Can you work these out from the drawing? Everything is in mm from the part's minimum corner. A direction names the side the tool comes from. Round coordinates to 2 decimals unless told otherwise and drop trailing zeros. Write each loop counter-clockwise with the first axis right and the second up, starting at its lowest first coordinate (ties: lowest second). Pieces come first, ordered by that corner, then holes. Notation, with made-up numbers: M 31.5,82.5 L 63.5,82.5 A13 cw 63.5,104.5 Z; hole C -30.5,-29 d5. An arc over 180 degrees is marked long. Answer in a Markdown table with one row per item. Add a question column.
(1) For the marked faces 1, 2 and 3, which set-ups out of +Z, -Z, +X, -X, +Y, -Y let a thin tool reach every point of the face, with its end or its side?
(2) I'm going to push flat-ended pins straight in: pin 1 (3 mm diameter, centred on x = 39.5, z = 11, fed in from +Y); pin 2 (1 mm diameter, centred on x = 37.5, y = 10, fed in from +Z); pin 3 (6 mm diameter, centred on y = 7.5, z = 44, fed in from +X). Where does each tip first touch, or does it pass through?
(3) Suppose I cut it at D-D, the plane y = 11.25. Count the separate pieces of the cut face and the enclosed holes in it, then the cut area to 3 significant figures.
(4) If we mould it in two halves opening along X, with no side actions, what happens to the marked faces 4, 5 and 6? For each: released by +X, released by -X, zero draft, split by the parting line, or undercut.
(5) Suppose I cut it at C-C, the plane x = 34.5. Write out the boundary of the cut face in (y, z) (1 decimal).
(6) If I drill on probe 1 along Z at (x, y) = (26, 8.5); probe 2 along Z at (x, y) = (36, 14) (1 decimal); probe 3 along Z at (x, y) = (41, 3) (1 decimal), over which ranges is the centre line in solid material (lowest first)?
(7) Suppose I cut it at B-B, the plane z = 26. Write out the boundary of the cut face in (x, y), then the cut area to 3 significant figures.
(8) Suppose I cut it at A-A, the plane x = 26. Write out the boundary of the cut face in (y, z), then the cut area to 3 significant figures.
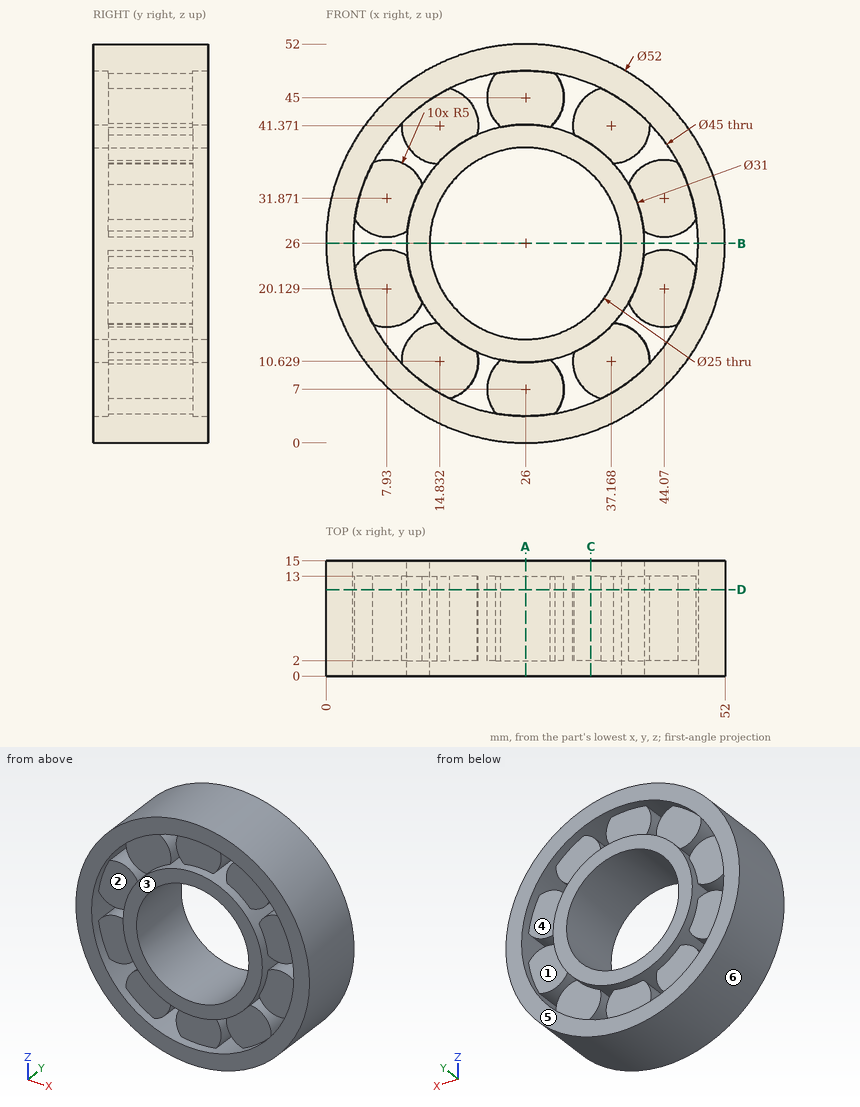
Calculated:
| question | item | result |
|---|---|---|
| 1 | face 1 | +Y |
| 1 | face 2 | -Y |
| 1 | face 3 | +Z, -Z, +X, -X, -Y |
| 2 | pin 1 | y = 13 |
| 2 | pin 2 | z = 49.56 |
| 2 | pin 3 | x = 47.24 |
| 3 | separate pieces | 1 |
| 3 | enclosed holes | 11 |
| 3 | area | 1,440 mm² |
| 4 | face 4 | undercut |
| 4 | face 5 | zero draft |
| 4 | face 6 | split by the parting line |
| 5 | outline | M 0,1.4 L 15,1.4 L 15,5.2 L 0,5.2 Z; M 0,13 L 2,13 L 2,6.4 L 13,6.4 L 13,13 L 15,13 L 15,16.8 L 0,16.8 Z; M 0,35.2 L 15,35.2 L 15,39 L 13,39 L 13,45.6 L 2,45.6 L 2,39 L 0,39 Z; M 0,46.8 L 15,46.8 L 15,50.6 L 0,50.6 Z |
| 6 | probe 1 | 0 to 13.5, 38.5 to 52 |
| 6 | probe 2 | 2 to 5.8, 14.2 to 18.5, 33.5 to 37.8, 46.2 to 50 |
| 6 | probe 3 | 4.8 to 13.8, 16.2 to 35.8, 38.2 to 47.2 |
| 7 | outline | M 0,0 L 3.5,0 L 3.5,15 L 0,15 Z; M 10.5,0 L 13.5,0 L 13.5,15 L 10.5,15 Z; M 38.5,0 L 41.5,0 L 41.5,15 L 38.5,15 Z; M 48.5,0 L 52,0 L 52,15 L 48.5,15 Z |
| 7 | area | 195 mm² |
| 8 | outline | M 0,0 L 15,0 L 15,3.5 L 13,3.5 L 13,10.5 L 15,10.5 L 15,13.5 L 0,13.5 L 0,10.5 L 2,10.5 L 2,3.5 L 0,3.5 Z; M 0,38.5 L 15,38.5 L 15,41.5 L 13,41.5 L 13,48.5 L 15,48.5 L 15,52 L 0,52 L 0,48.5 L 2,48.5 L 2,41.5 L 0,41.5 Z |
| 8 | area | 349 mm² |
